For this review, take the finished solid that the model builds, in its own axes (mm). Face numbers are marked on the shaded views. Give positions to 0.01 mm unless a question says otherwise; leave off trailing zeros. Order: outer loops, then holes, each group sorted by start corner. A loop starts at its lowest first (then second) coordinate and runs counter-clockwise, first axis right, second up. Notation, with made-up numbers: (-27, 68) -> (-1, 68) arc R19 cw to (-1, 85) -> close; hole circle Ø4 at (-15.75, 13). An arc over 180 degrees is marked (long way). Return JSON: item names as keys, results as strings. Group by question number.
1) Add section B-B (y = -12). Give the boundary of the cut face in (x, z), then the cut area to 3 significant figures.
2) Add section C-C (x = 12). Give the boundary of the cut face in (y, z).
3) To check wall thickness, follow line 1 along Y through (x, z) = (0, 5); line 2 along X through (y, z) = (-10, 5.5); line 3 along Y through (x, z) = (2, 1). State the ranges of each line that lie inside material, in increasing order.
4) The part is to be moulded in two halves that separate along Y. For the marked faces 1, 2, 3 and 4, say which applies: released by +Y, released by -Y, zero draft, split by the parting line, or undercut.
5) Add section A-A (z = 6). Give the boundary of the cut face in (x, y).
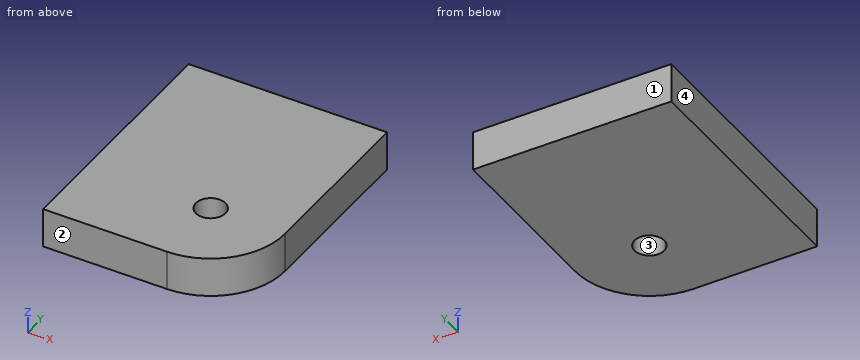
from build123d import *

# Parameters (mm, degrees)
F1_DEPTH = 8
F2_D     = 6


with BuildPart() as f1:
    # F0 (on Top) → F1 (new body)
    with BuildSketch(Plane.XY):
        with BuildLine():
            Line((15, -10), (15, 25))
            Line((15, 25), (-15, 25))
            Line((-15, 25), (-25, 25))
            Line((-25, 25), (-25, -25))
            Line((-25, -25), (-15, -25))
            Line((-15, -25), (0, -25))
            ThreePointArc((0, -25), (10.6066017178, -20.6066017178), (15, -10))
        make_face()
    extrude(amount=F1_DEPTH)

    # F2 (through all)
    with Locations(Plane(origin=(0, 0, 0), x_dir=(1, 0, 0), z_dir=(0, 0, -1))):
        with Locations((0, 10)):
            Hole(F2_D / 2)


solid = f1.part
Evaluation:
{
 "1": {"outline": "(-25, 0) -> (-2.24, 0) -> (-2.24, 8) -> (-25, 8) -> close; (2.24, 0) -> (14.87, 0) -> (14.87, 8) -> (2.24, 8) -> close", "area": "283 mm^2"},
 "2": {"outline": "(-19, 0) -> (25, 0) -> (25, 8) -> (-19, 8) -> close"},
 "3": {"line 1": "-25 to -13, -7 to 25", "line 2": "-25 to -3, 3 to 15", "line 3": "-24.87 to -12.24, -7.76 to 25"},
 "4": {"face 1": "released by +Y", "face 2": "released by -Y", "face 3": "undercut", "face 4": "zero draft"},
 "5": {"outline": "(-25, -25) -> (0, -25) arc R15 ccw to (15, -10) -> (15, 25) -> (-25, 25) -> close; hole circle Ø6 at (0, -10)"}
}
